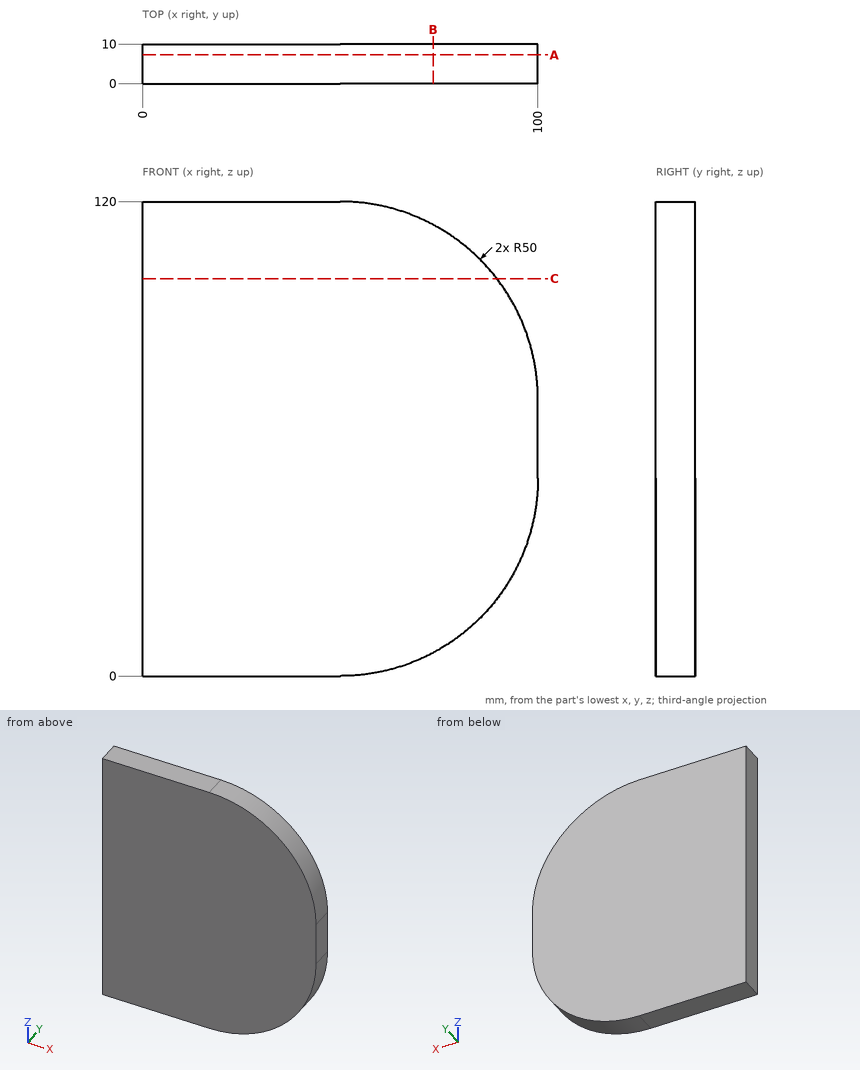
Can you work these out from the drawing? Everything is in mm from the part's minimum corner. Coordinates: 2 decimals unless noted, no trailing zeros. Write each loop counter-clockwise with the first axis right and the second up, starting at its lowest first coordinate (ties: lowest second). Pieces come first, ordered by that corner, then holes. Notation, with made-up numbers: (53, -39.75) - (97, -39.75) arc R23 ccw to (97, -5.75) - close; hole circle Ø1 at (-37, 27.25). An arc over 180 degrees is marked (long way). One line per item, written item: value.
1) Suppose I cut it at C-C on z = 100.5. Write out the boundary of the cut face in (x, y), and give its area (3 significant figures).
Model answer:
outline: (0, 0) - (89.62, 0) - (89.62, 10) - (0, 10) - close
area: 896 mm²
2) Suppose I cut it at A-A on y = 7.25. Write out the boundary of the cut face in (x, z), and give its area (3 significant figures).
Model answer:
outline: (0, 0) - (50, 0) arc R50 ccw to (100, 50) - (100, 70) arc R50 ccw to (50, 120) - (0, 120) - close
area: 10,900 mm²
3) I need wall thicknesses on line 1 along Z through (x, y) = (66, 3.25); line 2 along X through (y, z) = (4, 100.5); line 3 along Z through (x, y) = (88, 5.5). Which ranges of each line are inside material? Lowest first, please.
Model answer:
line 1: z = 2.63 to 117.37
line 2: x = 0 to 89.62
line 3: z = 17.5 to 102.5
4) Suppose I cut it at B-B on x = 73.5. Write out the boundary of the cut face in (y, z).
Model answer:
outline: (0, 5.87) - (10, 5.87) - (10, 114.13) - (0, 114.13) - close
5) I'm going to push flat-ended pins straight in: P1, Ø5, axis at y = 2.5, z = 16.5, coming from the +X side; P2, Ø6, axis at y = 4.5, z = 85.5, coming from the -X side; P3, Ø1.5, axis at x = 71.5, y = 6, coming from the -Z side; P4, Ø4, axis at y = 6, z = 101.5, coming from the +X side. Where does each tip first touch, or does it pass through?
Model answer:
P1: stops at x = 89.23
P2: stops at x = 0
P3: stops at z = 4.51
P4: stops at x = 90.37
